Design review of the part shown in the three views and the two pictorial views. Dimensions are in mm from the part's minimum x, y and z. A direction names the side the tool comes from. Coordinates: 2 decimals unless noted, no trailing zeros. Loops run counter-clockwise (first coordinate to the right, second up) from the corner with the lowest first, then second, coordinate; pieces in that order, holes last. Notation, with made-up numbers: M -11,-1.75 L 28,-1.75 A23 cw 28,35.25 Z; hole C -23,61.5 d8. An arc over 180 degrees is marked long. Put each result on its own line as item: value. Start each with the question number.
(1) The part is to be moulded in two halves that separate along Z. For the marked faces 3, 4, 5 and 6, say which applies: +Z half, -Z half, draft (parallel to the pull), parting line (faces both ways), or undercut.
(2) For probe 1 along X at (y, z) = (8.5, 14.5); probe 2 along Y at (x, z) = (8, 8), list the stretches that pass through material, from the lowest coordinate up. Write a range as [from, to].
(3) Take a section at A-A, the plane x = 12.5. Give the boundary of the cut face in (y, z), then the cut area to 3 significant figures.
(4) Take a section at C-C, the plane z = 2.5. Give the boundary of the cut face in (x, y), then the cut area to 3 significant figures.
(5) Take a section at B-B, the plane y = 7.75. Give the boundary of the cut face in (x, z).
(6) Clearance check with a flat-ended pin moving along its axis: pin 1 (4 mm diameter, centred on x = 8.5, z = 9, fed in from +Y). State where the tip first meets the part, or that it passes through.
(7) For the marked faces 1 and 2, list the 3-axis set-ups (+Z, -Z, +X, -X, +Y, -Y) from which the entire face can be reached by the end or side of a thin tool; tool diameter is ignored.
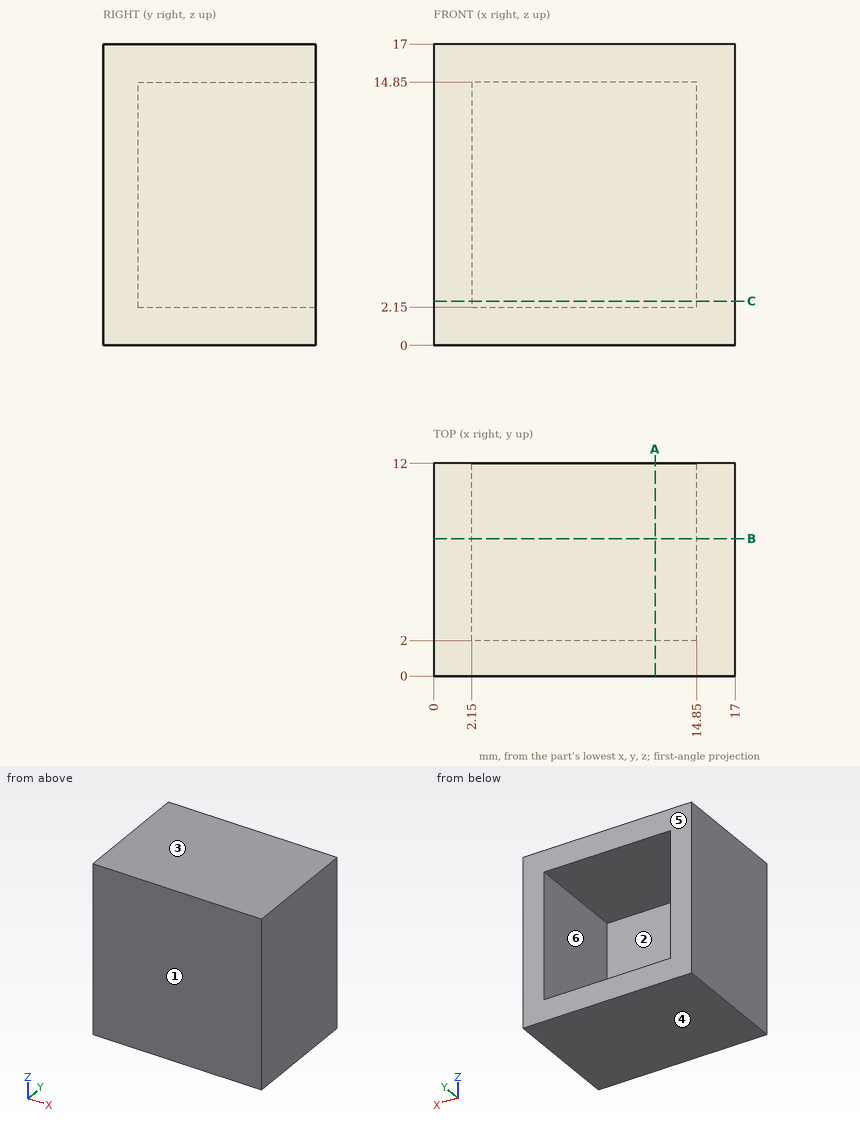
Computed values:
1. face 3: +Z half
1. face 4: -Z half
1. face 5: draft
1. face 6: undercut
2. probe 1: x = [0, 2.15], [14.85, 17]
2. probe 2: y = [0, 2]
3. outline: M 0,0 L 12,0 L 12,2.15 L 2,2.15 L 2,14.85 L 12,14.85 L 12,17 L 0,17 Z
3. area: 77.0 mm^2
4. outline: M 0,0 L 17,0 L 17,12 L 14.85,12 L 14.85,2 L 2.15,2 L 2.15,12 L 0,12 Z
4. area: 77.0 mm^2
5. outline: M 0,0 L 17,0 L 17,17 L 0,17 Z; hole M 2.15,2.15 L 14.85,2.15 L 14.85,14.85 L 2.15,14.85 Z
6. pin 1: stops at y = 2
7. face 1: +Z, -Z, +X, -X, -Y
7. face 2: +Y
